Here's how the part is built. I have some questions about the finished solid (model axes, mm). A direction names the side the tool comes from. Give positions to 0.01 mm unless a question says otherwise; leave off trailing zeros. Order: outer loops, then holes, each group sorted by start corner. A loop starts at its lowest first (then second) coordinate and runs counter-clockwise, first axis right, second up.
from build123d import *

# Parameters (mm, degrees)
BOSS_EXTRUDE1_DEPTH = 1
CUT_EXTRUDE2_DEPTH  = 84.653220646
CUT_EXTRUDE1_DEPTH  = 81.785527353
CHAMFER1_SIZE       = 1


with BuildPart() as part:
    # Sketch1 → Boss-Extrude1 (new body)
    with BuildSketch(Plane(origin=(0, 0, 0), x_dir=(1, 0, 0), z_dir=(0, 1, 0))):
        with BuildLine():
            Line((0, 49.519034561), (0, 59.764352058))
            ThreePointArc((0, 59.764352058), (37.735444373, 46.3445144), (58.524213344, 12.111739322))
            Line((58.524213344, 12.111739322), (48.491491054, 10.03544116))
            ThreePointArc((48.491491054, 10.03544116), (31.266511048, 38.399740504), (0, 49.519034561))
        make_face()
    extrude(amount=BOSS_EXTRUDE1_DEPTH)

    # Sketch3 → Cut-Extrude2 (cut, through all)
    with BuildSketch(Plane(origin=(0, 1, 0), x_dir=(1, 0, 0), z_dir=(0, 1, 0))):
        with BuildLine():
            ThreePointArc((0, 57.715288559), (36.441657708, 44.75555962), (56.517668886, 11.69647969))
            Line((56.517668886, 11.69647969), (58.524213344, 12.111739322))
            ThreePointArc((58.524213344, 12.111739322), (37.735444373, 46.3445144), (0, 59.764352058))
            Line((0, 59.764352058), (0, 57.715288559))
        make_face()
    extrude(amount=-CUT_EXTRUDE2_DEPTH, mode=Mode.SUBTRACT)

    # Sketch2 → Cut-Extrude1 (cut, through all)
    with BuildSketch(Plane(origin=(0, 1, 0), x_dir=(1, 0, 0), z_dir=(0, 1, 0))):
        Polygon((23.166733532, 49.681220385), (22.870900749, 49.046804934), (23.324054642, 48.835495803), (23.619887426, 49.469911254), align=None)
        Polygon((22.417746855, 49.258114065), (22.870900749, 49.046804934), (23.166733532, 49.681220385), (22.713579639, 49.892529516), align=None)
        Polygon((22.206437724, 48.804960172), (22.659591618, 48.593651041), (22.870900749, 49.046804934), (22.417746855, 49.258114065), align=None)
        Polygon((21.360713143, 48.647639061), (21.995128594, 48.351806278), (22.206437724, 48.804960172), (22.417746855, 49.258114065), (21.783331404, 49.553946848), align=None)
        Polygon((21.995128594, 48.351806278), (22.448282487, 48.140497147), (22.659591618, 48.593651041), (22.206437724, 48.804960172), align=None)
        Polygon((21.69929581, 47.717390827), (22.152449704, 47.506081696), (22.448282487, 48.140497147), (21.995128594, 48.351806278), align=None)
        Polygon((22.448282487, 48.140497147), (22.152449704, 47.506081696), (22.605603597, 47.294772565), (22.901436381, 47.929188016), align=None)
        Polygon((22.659591618, 48.593651041), (22.448282487, 48.140497147), (22.901436381, 47.929188016), (23.112745512, 48.38234191), align=None)
        Polygon((23.112745512, 48.38234191), (22.901436381, 47.929188016), (23.535851832, 47.633355233), (23.958470093, 48.53966302), (23.324054642, 48.835495803), align=None)
        Polygon((22.870900749, 49.046804934), (22.659591618, 48.593651041), (23.112745512, 48.38234191), (23.324054642, 48.835495803), align=None)
    extrude(amount=-CUT_EXTRUDE1_DEPTH, mode=Mode.SUBTRACT)

    # Chamfer1
    chamfer1_edges = [part.edges().sort_by_distance(p)[0] for p in [
        (21.847212202, 1, -48.034598553),
        (22.152449704, 1, -47.506081696),
        (22.753519989, 1, -47.611980291),
        (23.218644106, 1, -47.781271625),
        (23.747160962, 1, -48.086509127),
        (23.641262368, 1, -48.687579412),
        (23.471971034, 1, -49.152703529),
        (23.166733532, 1, -49.681220385),
        (22.565663247, 1, -49.575321791),
        (22.10053913, 1, -49.406030457),
        (21.572022274, 1, -49.100792955),
        (21.677920868, 1, -48.49972267),
    ]]
    chamfer(chamfer1_edges, length=CHAMFER1_SIZE - 0.0001)  # a hair under: the kernel refuses the full size


solid = part.part
Q1. For faces 4 (the face through (33, 0, -38)), 5 (the face through (23.5, 0.5, -47.1)), which set-ups out of +Z, -Z, +X, -X, +Y, -Y let a thin tool reach every point of the face, with its end or its side?
Filled sheet:
face 4: +Z, -Z, +X, -X, -Y
face 5: +Y
Q2. If we section it at A-A on y = 0.35: List the corners of the cut face in (x, z) for me.
Filled sheet:
outline: (0, -57.72) arc R57.72 ccw to (56.52, -11.7) - (48.49, -10.04) arc R49.52 cw to (0, -49.52) - close; hole (20.9, -48.48) - (21.61, -50.02) - (22.25, -49.72) - (22.54, -50.36) - (24.08, -49.64) - (23.79, -49) - (24.42, -48.71) - (23.71, -47.17) - (23.07, -47.46) - (22.77, -46.83) - (21.23, -47.55) - (21.53, -48.18) - close
Q3. If we section it at B-B on x = 19: List the corners of the cut face in (y, z) for me, plus the area to 3 significant figures.
Filled sheet:
outline: (0, -54.5) - (1, -54.5) - (1, -45.73) - (0, -45.73) - close
area: 8.77 mm2
Q4. I'm going to push a flat-ended pin straight in: P1, Ø8, axis at x = 42, z = -50.5, coming from the -Y side. Where does the tip first touch, or does it pass through?
Filled sheet:
P1: passes through
Q5. Thinking about a two-plate mould opening in Z: for faces 1 (the face through (31.63, 0.49, -38.1)), 2 (the face through (36.012, 0.507, -45.102)), 3 (the face through (21.867, 0.493, -50.059)), which applies, released by +Z, released by -Z, zero draft, split by the parting line, or undercut?
Filled sheet:
face 1: released by +Z
face 2: released by -Z
face 3: undercut
Q6. If we section it at C-C on z = -21: List the corners of the cut face in (x, y) for me, plus the area to 3 significant figures.
Filled sheet:
outline: (44.85, 0) - (53.76, 0) - (53.76, 1) - (44.85, 1) - close
area: 8.91 mm2
Q7. I need wall thicknesses on L1, parallel to Z at x = 52, y = 0.75; L2, parallel to Z at x = 39, y = 0.7; L3, parallel to X at y = 0.5, z = -38.5. Which ranges of each line are inside material? Lowest first, please.
Filled sheet:
L1: z = -25.04 to -10.76
L2: z = -42.54 to -30.51
L3: x = 31.14 to 43
